Design review of the part built by this model. Coordinates are the model's own, in mm. Face numbers are marked on the shaded views. A direction names the side the tool comes from. Coordinates: 2 decimals unless noted, no trailing zeros. Write each loop counter-clockwise with the first axis right and the second up, starting at its lowest first coordinate (ties: lowest second). Pieces come first, ordered by that corner, then holes. Notation, with made-up numbers: (-14, 56.5) - (12, 56.5) arc R25 ccw to (12, 68.5) - close; hole circle Ø10 at (54, 25.25). An arc over 180 degrees is marked (long way). One line per item, written item: value.
from build123d import *

# Parameters (mm, degrees)
SKETCH_1_W          = 13
SKETCH_1_H          = 13
EXTRUDE_1_DEPTH     = 1.1
SKETCH_2_W          = 4.3
SKETCH_2_H          = 5
EXTRUDE_2_DEPTH     = 1
SKETCH_3_W          = 2.1
SKETCH_3_H          = 1.3
EXTRUDE_3_DEPTH     = 0.8
SKETCH_4_W          = 1
SKETCH_4_H          = 1.5
EXTRUDE_4_DEPTH     = 0.1
SKETCH_5_R          = 1
CUT_EXTRUDE_1_DEPTH = 1.1


with BuildPart() as part:
    # 스케치1 → 보스-돌출1 (new body)
    with BuildSketch(Plane.XY):
        Rectangle(SKETCH_1_W, SKETCH_1_H)
    extrude(amount=EXTRUDE_1_DEPTH)

    # 스케치2 → 보스-돌출2 (add)
    with BuildSketch(Plane.XY.offset(1.1)):
        Rectangle(SKETCH_2_W, SKETCH_2_H)
    extrude(amount=EXTRUDE_2_DEPTH)

    # 스케치3 → 보스-돌출3 (add)
    with BuildSketch(Plane.XY.offset(1.1)):
        with Locations((-2.05, 4.5)):
            Rectangle(SKETCH_3_W, SKETCH_3_H)
        with Locations((2.05, 4.5)):
            Rectangle(SKETCH_3_W, SKETCH_3_H)
    extrude(amount=EXTRUDE_3_DEPTH)

    # 스케치4 → 보스-돌출4 (add)
    with BuildSketch(Plane.XY.offset(1.1)):
        with Locations((-2.91, -4.75)):
            Rectangle(SKETCH_4_W, SKETCH_4_H)
        with Locations((4.85, -4.75)):
            Rectangle(SKETCH_4_W, SKETCH_4_H)
        with Locations((-4.85, -4.75)):
            Rectangle(SKETCH_4_W, SKETCH_4_H)
        with Locations((-0.97, -4.75)):
            Rectangle(SKETCH_4_W, SKETCH_4_H)
        with Locations((0.97, -4.75)):
            Rectangle(SKETCH_4_W, SKETCH_4_H)
        with Locations((2.91, -4.75)):
            Rectangle(SKETCH_4_W, SKETCH_4_H)
    extrude(amount=EXTRUDE_4_DEPTH)

    # 스케치5 → 컷-돌출1 (cut)
    with BuildSketch(Plane.XY.offset(1.1)):
        with Locations((5.6, 0)):
            Circle(SKETCH_5_R)
        with Locations((-5.6, 0)):
            Circle(SKETCH_5_R)
    extrude(amount=-CUT_EXTRUDE_1_DEPTH, mode=Mode.SUBTRACT)


solid = part.part
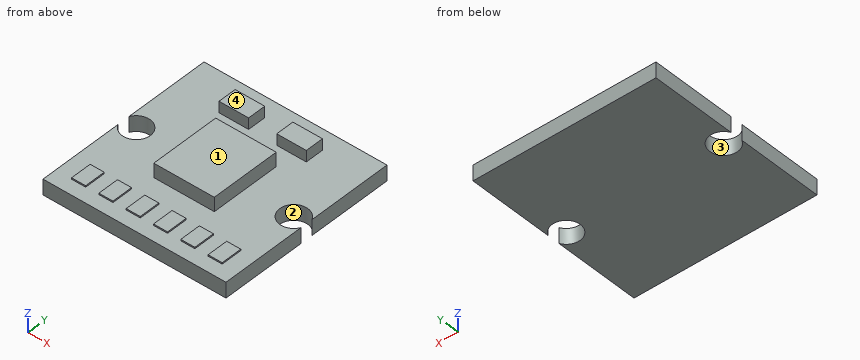
1. Consider section B-B, the plane x = 5.6. Write out the cut boundary in (y, z).
Answer block:
outline: (-6.5, 0) - (-1, 0) - (-1, 1.1) - (-6.5, 1.1) - close; (1, 0) - (6.5, 0) - (6.5, 1.1) - (1, 1.1) - close
2. Wall thickness on line 1 along Y through (x, z) = (5.6, 0.5); line 2 along Y through (x, z) = (1.75, 1.7); line 3 along Z through (x, y) = (-5.25, 3.5): over which ranges is each line inside the solid? List them lowest first.
Answer block:
line 1: y = -6.5 to -1, 1 to 6.5
line 2: y = -2.5 to 2.5, 3.85 to 5.15
line 3: z = 0 to 1.1
3. For the marked faces 3 and 4, list the 3-axis set-ups (+Z, -Z, +X, -X, +Y, -Y) from which the entire face can be reached by the end or side of a thin tool; tool diameter is ignored.
Answer block:
face 3: +Z, -Z
face 4: +Z, +X, -X, +Y
4. Consider section C-C, the plane y = 0. Write out the cut boundary in (x, z).
Answer block:
outline: (-4.6, 0) - (4.6, 0) - (4.6, 1.1) - (2.15, 1.1) - (2.15, 2.1) - (-2.15, 2.1) - (-2.15, 1.1) - (-4.6, 1.1) - close
5. Consider section A-A, the plane z = 1.4. Write out the cut boundary in (x, y).
Answer block:
outline: (-3.1, 3.85) - (-1, 3.85) - (-1, 5.15) - (-3.1, 5.15) - close; (-2.15, -2.5) - (2.15, -2.5) - (2.15, 2.5) - (-2.15, 2.5) - close; (1, 3.85) - (3.1, 3.85) - (3.1, 5.15) - (1, 5.15) - close
6. Mouldability with a two-part tool opening along Y and no side actions: class the marked faces 1 and 2 as released by +Y, released by -Y, zero draft, split by the parting line, or undercut.
Answer block:
face 1: zero draft
face 2: undercut
7. Insertion check: pin 1 Ø1.1 at (x, z) = (0.5, 2) entering from +Y; pin 2 Ø0.8 at (y, z) = (0.5, 2) entering from -X; pin 3 Ø0.8 at (x, y) = (-1, -4.5) entering from +Z. Each pin has a flat end and moves straight along its axis. Give the tip position at first contact, or say it passes through.
Answer block:
pin 1: stops at y = 5.15
pin 2: stops at x = -2.15
pin 3: stops at z = 1.2
8. Consider section D-D, the plane x = -0.25. Write out the cut boundary in (y, z), then the cut area to 3 significant figures.
Answer block:
outline: (-6.5, 0) - (6.5, 0) - (6.5, 1.1) - (2.5, 1.1) - (2.5, 2.1) - (-2.5, 2.1) - (-2.5, 1.1) - (-6.5, 1.1) - close
area: 19.3 mm^2
